Geometry check sheet. Reference: the model listing, model coordinates, mm. Face numbers are marked on the shaded views. A direction names the side the tool comes from. Round coordinates to 2 decimals unless told otherwise and drop trailing zeros. Write each loop counter-clockwise with the first axis right and the second up, starting at its lowest first coordinate (ties: lowest second). Pieces come first, ordered by that corner, then holes. Notation, with made-up numbers: (-37.5, 76) -> (21.5, 76) arc R23 ccw to (21.5, 100) -> close; hole circle Ø2 at (88.5, 65.25). An arc over 180 degrees is marked (long way). Use a Markdown table: item, result.
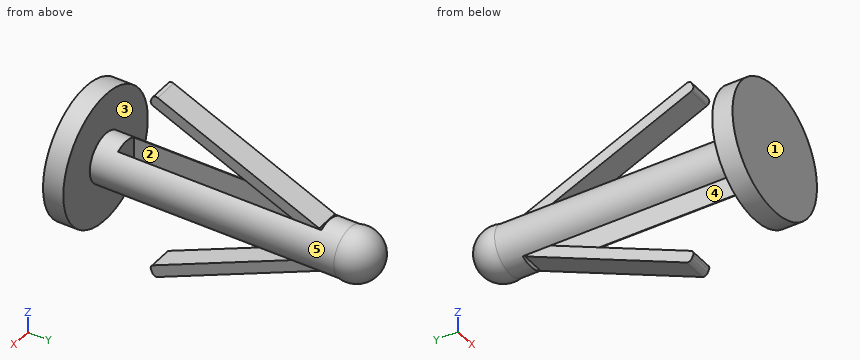
```python
from build123d import *

# Parameters (mm, degrees)
SKETCH1_R               = 16
BOSS_EXTRUDE1_DEPTH     = 5
SKETCH2_R               = 6
BOSS_EXTRUDE2_DEPTH     = 60
DOME1_FACE_RADIUS       = 6
DOME1_HEIGHT            = 8
SKETCH3_W               = 6
SKETCH3_H               = 50
CUT_EXTRUDE1_DEPTH      = 6
CUT_EXTRUDE1_DEPTH_BACK = 6
BOSS_EXTRUDE6_DEPTH     = 6
FILLET2_R               = 1
FILLET4_R               = 1
FILLET2_OF_MIRROR2_R    = 1
FILLET4_OF_MIRROR2_R    = 1


with BuildPart() as part:
    # Sketch1 → Boss-Extrude1 (new body)
    with BuildSketch(Plane(origin=(0, 0, 0), x_dir=(1, 0, 0), z_dir=(0, 1, 0))):
        Circle(SKETCH1_R)
    extrude(amount=-BOSS_EXTRUDE1_DEPTH)

    # Sketch2 → Boss-Extrude2 (add)
    with BuildSketch(Plane(origin=(0, 0, 0), x_dir=(1, 0, 0), z_dir=(0, 1, 0))):
        Circle(SKETCH2_R)
    extrude(amount=BOSS_EXTRUDE2_DEPTH)

    # Dome1: a dome of height H over a round flat face of radius A is a cap of a sphere of radius (A * A + H * H) / (2 * H)
    dome1_r = (DOME1_FACE_RADIUS * DOME1_FACE_RADIUS + DOME1_HEIGHT * DOME1_HEIGHT) / (2 * DOME1_HEIGHT)
    dome1_base = Plane((0, 60, 0), z_dir=(0, 1, 0))
    with Locations(dome1_base.offset(DOME1_HEIGHT - dome1_r)):
        dome1_ball = Sphere(dome1_r, mode=Mode.PRIVATE)
    add(split(dome1_ball, bisect_by=dome1_base, keep=Keep.TOP, mode=Mode.PRIVATE))

    # Sketch3 → Cut-Extrude1 (cut, two sides)
    with BuildSketch(Plane.XY) as cut_extrude1_sk:
        with Locations((-0.023759129, 30)):
            Rectangle(SKETCH3_W, SKETCH3_H)
    extrude(amount=CUT_EXTRUDE1_DEPTH, mode=Mode.SUBTRACT)
    extrude(cut_extrude1_sk.sketch, amount=-CUT_EXTRUDE1_DEPTH_BACK, mode=Mode.SUBTRACT)

    # Sketch4 → Boss-Extrude6 (add)
    with BuildSketch(Plane.ZY.offset(-2.976240871)):
        Polygon((5.454631491, 54.445098747), (23.375133838, 13.829372646), (20.834979102, 12.708603592), (2.914476754, 53.324329693), align=None)
    boss_extrude6 = extrude(amount=BOSS_EXTRUDE6_DEPTH)

    # Fillet2
    fillet2_edges = [part.edges().sort_by_distance(p)[0] for p in [
        (-0.023759129, 13.829372646, 23.375133838),
    ]]
    fillet(fillet2_edges, radius=FILLET2_R)

    # Fillet4
    fillet4_edges = [part.edges().sort_by_distance(p)[0] for p in [
        (-0.023759129, 12.708603592, 20.834979102),
    ]]
    fillet(fillet4_edges, radius=FILLET4_R)

    # Mirror2: Boss-Extrude6 across plane
    add(boss_extrude6.mirror(Plane.XY))

    # Fillet2 of Mirror2
    fillet2_of_mirror2_edges = [part.edges().sort_by_distance(p)[0] for p in [
        (-0.023759129, 13.829372646, -23.375133838),
    ]]
    fillet(fillet2_of_mirror2_edges, radius=FILLET2_OF_MIRROR2_R)

    # Fillet4 of Mirror2
    fillet4_of_mirror2_edges = [part.edges().sort_by_distance(p)[0] for p in [
        (-0.023759129, 12.708603592, -20.834979102),
    ]]
    fillet(fillet4_of_mirror2_edges, radius=FILLET4_OF_MIRROR2_R)


solid = part.part
```
(1) Section check A-A on x = 0. Record the cut outline in (y, z), plus the area to 3 significant figures.
A:
| item | result |
|---|---|
| outline | (-5, -16) -> (0, -16) -> (0, -6) -> (5, -6) -> (5, 6) -> (0, 6) -> (0, 16) -> (-5, 16) -> close; (13.11, -21.75) -> (13.43, -22.46) arc R1 ccw to (14.74, -22.97) -> (54.45, -5.45) -> (53.32, -2.91) -> (13.62, -20.43) arc R1 ccw to start; (13.11, 21.75) arc R1 ccw to (13.62, 20.43) -> (53.32, 2.91) -> (54.45, 5.45) -> (14.74, 22.97) arc R1 ccw to (13.43, 22.46) -> close; (55, -6) -> (60, -6) arc R6.25 ccw (long way) to (60, 6) -> (55, 6) -> close |
| area | 609 mm2 |
(2) Access from +Z, -Z, +X, -X, +Y, -Y to the whole of each face (thin tool, end or side, straight path). Record for the marked faces 1 and 2.
A:
| item | result |
|---|---|
| face 1 | +Z, -Z, +X, -X, -Y |
| face 2 | none |
(3) Section check B-B on z = 0. Record the cut outline in (x, y).
A:
| item | result |
|---|---|
| outline | (-16, -5) -> (16, -5) -> (16, 0) -> (6, 0) -> (6, 60) arc R6.25 ccw (long way) to (-6, 60) -> (-6, 0) -> (-16, 0) -> close; hole (-3.02, 5) -> (2.98, 5) -> (2.98, 55) -> (-3.02, 55) -> close |
(4) Thickness scan on line 1 (Y direction, x = -4, z = -14); line 2 (Y direction, x = 1, z = 7.5); line 3 (Y direction, x = 1, z = 0.5). Record the ranges inside material, lowest first.
A:
| item | result |
|---|---|
| line 1 | y = -5 to 0 |
| line 2 | y = -5 to 0, 42.93 to 49.81 |
| line 3 | y = -5 to 5, 55 to 67.9 |
(5) Section check D-D on x = 4.5. Record the cut outline in (y, z), plus the area to 3 significant figures.
A:
| item | result |
|---|---|
| outline | (-5, -15.35) -> (0, -15.35) -> (0, -3.97) -> (60, -3.97) arc R4.34 ccw (long way) to (60, 3.97) -> (0, 3.97) -> (0, 15.35) -> (-5, 15.35) -> close |
| area | 674 mm2 |
(6) Gauge pin test, flat ends, axial feed: pin 1 Ø3 at (y, z) = (21, 3) entering from +X; pin 2 Ø1 at (x, z) = (3, 2.5) entering from +Y; pin 3 Ø5 at (y, z) = (19.5, 1.5) entering from -X. Record the tip position at first contact, or that the pin passes through.
A:
| item | result |
|---|---|
| pin 1 | stops at x = 5.81 |
| pin 2 | stops at y = 66.99 |
| pin 3 | stops at x = -6 |
(7) Section check C-C on y = 6.5. Record the cut outline in (x, z).
A:
| item | result |
|---|---|
| outline | (-3.02, -5.18) -> (-3.02, 5.18) arc R6 ccw to start; (2.98, -5.21) arc R6 ccw to (2.98, 5.21) -> close |
(8) Release check for a two-part mould opening along Z. For the marked faces 3, 4 and 5 record: +Z half, -Z half, draft (parallel to the pull), parting line (faces both ways), or undercut.
A:
| item | result |
|---|---|
| face 3 | draft |
| face 4 | undercut |
| face 5 | parting line |
